from build123d import *

# Parameters (mm, degrees)
SKETCH_1_W           = 220
SKETCH_1_H           = 70
EXTRUDE_1_DEPTH      = 3
EXTRUDE_2_DEPTH      = 25
EXTRUDE_2_DEPTH_BACK = 25
SKETCH_6_W           = 30
SKETCH_6_H           = 37.527767497
CUT_EXTRUDE_4_DEPTH  = 221
SKETCH_7_R           = 35
CUT_EXTRUDE_5_DEPTH  = 4
SKETCH_8_W           = 3
SKETCH_8_H           = 40
EXTRUDE_3_DEPTH      = 65
SKETCH_9_R           = 1.5
CUT_EXTRUDE_6_DEPTH  = 4
FILLET_5_R           = 1
SKETCH_12_R          = 1.5
CUT_EXTRUDE_8_DEPTH  = 4


with BuildPart() as part:
    # 草图1 → 凸台-拉伸1 (new body)
    with BuildSketch(Plane(origin=(0, 0, 0), x_dir=(1, 0, 0), z_dir=(0, 1, 0))):
        with Locations((27.295373665, 0)):
            Rectangle(SKETCH_1_W, SKETCH_1_H)
    extrude(amount=EXTRUDE_1_DEPTH)

    # 草图2 → 凸台-拉伸2 (add, two sides)
    with BuildSketch(Plane.XY) as extrude_2_sk:
        Polygon((-82.704626335, 40.527767497), (-82.704626335, 3), (-17.704626335, 3), align=None)
    extrude(amount=EXTRUDE_2_DEPTH)
    extrude(extrude_2_sk.sketch, amount=-EXTRUDE_2_DEPTH_BACK)

    # 草图6 → 切除-拉伸4 (cut, through all)
    with BuildSketch(Plane.ZY.offset(82.704626335)):
        with Locations((0, 21.763883748)):
            Rectangle(SKETCH_6_W, SKETCH_6_H)
    extrude(amount=-CUT_EXTRUDE_4_DEPTH, mode=Mode.SUBTRACT)

    # 草图7 → 切除-拉伸5 (cut, through all)
    with BuildSketch(Plane(origin=(0, 3, 0), x_dir=(1, 0, 0), z_dir=(0, 1, 0))):
        with Locations((25.295373665, 51)):
            Circle(SKETCH_7_R)
        with Locations((25.295373665, -51)):
            Circle(SKETCH_7_R)
    extrude(amount=-CUT_EXTRUDE_5_DEPTH, mode=Mode.SUBTRACT)

    # 草图8 → 凸台-拉伸3 (add)
    with BuildSketch(Plane.ZY.offset(82.704626335)):
        with Locations((36.5, 20)):
            Rectangle(SKETCH_8_W, SKETCH_8_H)
        with Locations((-36.5, 20)):
            Rectangle(SKETCH_8_W, SKETCH_8_H)
    extrude(amount=-EXTRUDE_3_DEPTH)

    # 草图9 → 切除-拉伸6 (cut, through all)
    with BuildSketch(Plane(origin=(0, 3, 0), x_dir=(1, 0, 0), z_dir=(0, 1, 0))):
        with Locations((-74.766784803, 29.860059225)):
            Circle(SKETCH_9_R)
        with Locations((-54.766784803, 29.860059225)):
            Circle(SKETCH_9_R)
        with Locations((-34.766784803, 29.860059225)):
            Circle(SKETCH_9_R)
        with Locations((-34.766784803, -29.860059225)):
            Circle(SKETCH_9_R)
        with Locations((-54.766784803, -29.860059225)):
            Circle(SKETCH_9_R)
        with Locations((-74.766784803, -29.860059225)):
            Circle(SKETCH_9_R)
        with Locations((68.031562246, 22)):
            Circle(SKETCH_9_R)
        with Locations((88.031562246, 22)):
            Circle(SKETCH_9_R)
        with Locations((108.031562246, 22)):
            Circle(SKETCH_9_R)
        with Locations((108.031562246, -22)):
            Circle(SKETCH_9_R)
        with Locations((88.031562246, -22)):
            Circle(SKETCH_9_R)
        with Locations((68.031562246, -22)):
            Circle(SKETCH_9_R)
        with Locations((128.031562246, 22)):
            Circle(SKETCH_9_R)
        with Locations((128.031562246, -22)):
            Circle(SKETCH_9_R)
    extrude(amount=-CUT_EXTRUDE_6_DEPTH, mode=Mode.SUBTRACT)

    # 圆角5
    fillet_5_edges = [part.edges().sort_by_distance(p)[0] for p in [
        (-50.204626335, 21.763883749, -25),
        (-50.204626335, 21.763883749, 25),
        (-50.204626335, 21.763883749, -15),
        (-50.204626335, 21.763883749, 15),
    ]]
    fillet(fillet_5_edges, radius=FILLET_5_R)

    # 草图12 → 切除-拉伸8 (cut, through all)
    with BuildSketch(Plane(origin=(0, 3, 0), x_dir=(1, 0, 0), z_dir=(0, 1, 0))):
        with BuildLine():
            Line((51.424138498, 27.712929589), (51.424138498, 0))
            Line((51.424138498, 0), (51.424138498, -27.712929589))
            ThreePointArc((51.424138498, -27.712929589), (54.155060508, -31.198018398), (56.424138498, -35))
            Line((56.424138498, -35), (137.295373665, -35))
            Line((137.295373665, -35), (137.295373665, 35))
            Line((137.295373665, 35), (56.424138498, 35))
            ThreePointArc((56.424138498, 35), (54.155060508, 31.198018398), (51.424138498, 27.712929589))
        make_face()
        with Locations((68.031562246, -22)):
            Circle(SKETCH_12_R, mode=Mode.SUBTRACT)
        with Locations((88.031562246, -22)):
            Circle(SKETCH_12_R, mode=Mode.SUBTRACT)
        with Locations((108.031562246, -22)):
            Circle(SKETCH_12_R, mode=Mode.SUBTRACT)
        with Locations((128.031562246, -22)):
            Circle(SKETCH_12_R, mode=Mode.SUBTRACT)
        with Locations((68.031562246, 22)):
            Circle(SKETCH_12_R, mode=Mode.SUBTRACT)
        with Locations((88.031562246, 22)):
            Circle(SKETCH_12_R, mode=Mode.SUBTRACT)
        with Locations((108.031562246, 22)):
            Circle(SKETCH_12_R, mode=Mode.SUBTRACT)
        with Locations((128.031562246, 22)):
            Circle(SKETCH_12_R, mode=Mode.SUBTRACT)
    extrude(amount=-CUT_EXTRUDE_8_DEPTH, mode=Mode.SUBTRACT)


solid = part.part
The listing builds one solid part. Answer for the finished solid, in the listing's coordinates (mm). A direction names the side the tool comes from. Round coordinates to 2 decimals unless told otherwise and drop trailing zeros. Order: outer loops, then holes, each group sorted by start corner. A loop starts at its lowest first (then second) coordinate and runs counter-clockwise, first axis right, second up. Notation, with made-up numbers: M 51,0.5 L 66,0.5 A22 ccw 66,34.5 Z; hole C 55,85.5 d3. An arc over 180 degrees is marked long. Answer in a Markdown table with one row per item. Add a question column.
1) Determine the mould class of faces 5 (the face through (-49.9, 21.241, -15.285)), 6 (the face through (-74.07, 1.52, 31.19)), 7 (the face through (-31, 0, -1)) for opening direction X: pulls with the +X half, pulls with the -X half, needs draft (parallel to the pull), parting line crosses it, or undercut.
2) The part is cut by section B-B on y = 30. Count the separate pieces of the cut face and the enclosed holes in it, plus the area to 3 significant figures.
3) Which of the six approach directions +Z, -Z, +X, -X, +Y, -Y give full straight-line access (tool end or side, diameter ignored) to faces 1 (the face through (20.406, 1.521, -16.343)), 2 (the face through (-12, 1, -35)), 3 (the face through (-49.75, 21.5, 20.06)), 4 (the face through (-59, 17, 15))?
4) The part is cut by section C-C on x = 27.5. Determine the outline of the cut face in (y, z).
5) The part is cut by section D-D on z = -5. Determine the outline of the cut face in (x, y).
6) Flat-ended cylindrical pins translate along their axes: pin 1 Ø10 at (x, y) = (31.5, 4) entering from +Z; pin 2 Ø5 at (x, z) = (-54.77, -29.86) entering from +Y; pin 3 Ø0.9 at (x, z) = (-63, 37) entering from +Y; pin 4 Ø2.5 at (x, z) = (-54.77, 29.86) entering from -Y. Find the tip coordinate at first contact, or state that the pin passes through.
7) The part is cut by section A-A on z = -22.5. Determine the outline of the cut face in (x, y), plus the area to 3 significant figures.
8) Consider line 1 along Z through (x, y) = (-39, 3.5); line 2 along Z through (x, y) = (-26, 32.5); line 3 along Y through (x, z) = (-56, 7). Determine where each line is inside the solid, lowest interval first. Write a range as from..to.
Findings below:
| question | item | result |
|---|---|---|
| 1 | face 5 | pulls with the +X half |
| 1 | face 6 | undercut |
| 1 | face 7 | needs draft |
| 2 | separate pieces | 4 |
| 2 | enclosed holes | 0 |
| 2 | area | 753 mm² |
| 3 | face 1 | -Z, +Y, -Y |
| 3 | face 2 | -Z, +X, +Y, -Y |
| 3 | face 3 | +X, +Y |
| 3 | face 4 | +X, -X, +Y |
| 4 | outline | M 0,-16.07 L 3,-16.07 L 3,16.07 L 0,16.07 Z |
| 5 | outline | M -82.7,0 L 51.42,0 L 51.42,3 L -82.7,3 Z |
| 6 | pin 1 | stops at z = 17.81 |
| 6 | pin 2 | stops at y = 3 |
| 6 | pin 3 | stops at y = 40 |
| 6 | pin 4 | passes through |
| 7 | outline | M -82.7,0 L 4.98,0 L 4.98,3 L -17.7,3 L -82.7,40.53 Z; M 45.61,0 L 51.42,0 L 51.42,3 L 45.61,3 Z |
| 7 | area | 1,500 mm² |
| 8 | line 1 | z = -38..-35, -25..-15, 15..25, 35..38 |
| 8 | line 2 | z = -38..-35, 35..38 |
| 8 | line 3 | y = 0..3 |
